```python
from build123d import *

# Parameters (mm, degrees)
EXTRUDE_1_DEPTH     = 120
CUT_EXTRUDE_1_DEPTH = 50
SKETCH_3_R          = 5
CUT_EXTRUDE_2_DEPTH = 10


with BuildPart() as part:
    # Эскиз1 → Вытянуть-Тонкостенный1 (new body)
    with BuildSketch(Plane(origin=(0, 0, 0), x_dir=(0, 0, -1), z_dir=(1, 0, 0))):
        Polygon((0, 40), (0, 0), (40, 0), (40, -3), (-3, -3), (-3, 40), align=None)
    extrude(amount=EXTRUDE_1_DEPTH)

    # Эскиз2 → Вырез-Вытянуть1 (cut)
    with BuildSketch(Plane(origin=(0, -3, 0), x_dir=(1, 0, 0), z_dir=(0, 1, 0))):
        Polygon((0, 40), (20, -3), (0, -3), align=None)
    extrude(amount=CUT_EXTRUDE_1_DEPTH, mode=Mode.SUBTRACT)

    # Эскиз3 → Вырез-Вытянуть2 (cut)
    with BuildSketch(Plane.XY.offset(3)):
        with Locations((70, 15)):
            Circle(SKETCH_3_R)
    extrude(amount=-CUT_EXTRUDE_2_DEPTH, mode=Mode.SUBTRACT)


solid = part.part
```
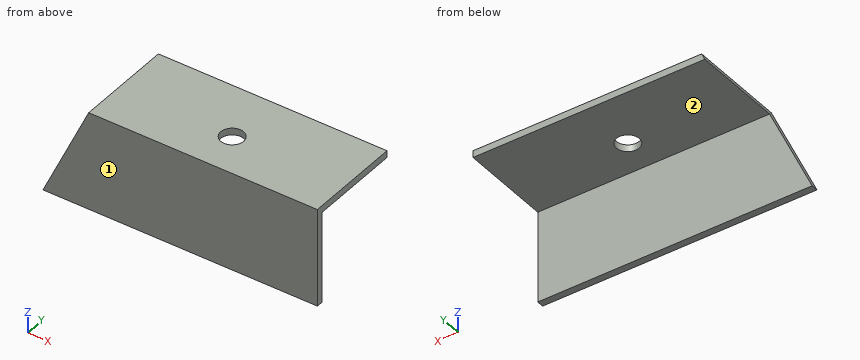
The listing builds one solid part. Answer for the finished solid, in the listing's coordinates (mm). Face numbers are marked on the shaded views. A direction names the side the tool comes from. Coordinates: 2 decimals unless noted, no trailing zeros. Loops run counter-clockwise (first coordinate to the right, second up) from the corner with the lowest first, then second, coordinate; pieces in that order, holes last. Notation, with made-up numbers: (17.5, -32) - (46.5, -32) arc R22 ccw to (46.5, -18) - close; hole circle Ø3 at (46, 78). An arc over 180 degrees is marked (long way). Use a Markdown table: item, result. Add a question column.
1) The part is cut by section C-C, the plane y = 24.5. Give the vertices of the cut face in (x, z), and give its area (3 significant figures).
2) Given pin 1 (1 mm diameter, centred on x = 81, y = 21, fed in from -Z); pin 2 (20 mm diameter, centred on x = 88.5, z = -22.5, fed in from +Y), each flat-ended and moving along its own axis, determine where each tip first touches the part or whether it passes through.
3) Find the intervals of material crossed by line 1 (Y direction, x = 70, z = 1.1); line 2 (Z direction, x = 100, y = 29.5); line 3 (Y direction, x = 40.5, z = -3.5), in increasing order.
4) For the marked faces 1 and 2, determine the directions among +Z, -Z, +X, -X, +Y, -Y from which every point of the face is accessible in a straight line to the end or side of a thin tool.
5) The part is cut by section D-D, the plane z = -35. Give the vertices of the cut face in (x, y), and give its area (3 significant figures).
6) The part is cut by section B-B, the plane y = 15. Give the vertices of the cut face in (x, z), and give its area (3 significant figures).
7) The part is cut by section A-A, the plane x = 70. Give the vertices of the cut face in (y, z).
Here are the results:
| question | item | result |
|---|---|---|
| 1 | outline | (18.6, 0) - (120, 0) - (120, 3) - (20, 3) - close |
| 1 | area | 302 mm^2 |
| 2 | pin 1 | stops at z = 0 |
| 2 | pin 2 | stops at y = 0 |
| 3 | line 1 | y = -3 to 10, 20 to 40 |
| 3 | line 2 | z = 0 to 3 |
| 3 | line 3 | y = -3 to 0 |
| 4 | face 1 | +Z, -Z, +X, -X, -Y |
| 4 | face 2 | -Z, +X, -X, +Y |
| 5 | outline | (2.33, -3) - (120, -3) - (120, 0) - (2.33, 0) - close |
| 5 | area | 353 mm^2 |
| 6 | outline | (18.6, 0) - (65, 0) - (65, 3) - (20, 3) - close; (75, 0) - (120, 0) - (120, 3) - (75, 3) - close |
| 6 | area | 272 mm^2 |
| 7 | outline | (-3, -40) - (0, -40) - (0, 0) - (10, 0) - (10, 3) - (-3, 3) - close; (20, 0) - (40, 0) - (40, 3) - (20, 3) - close |
